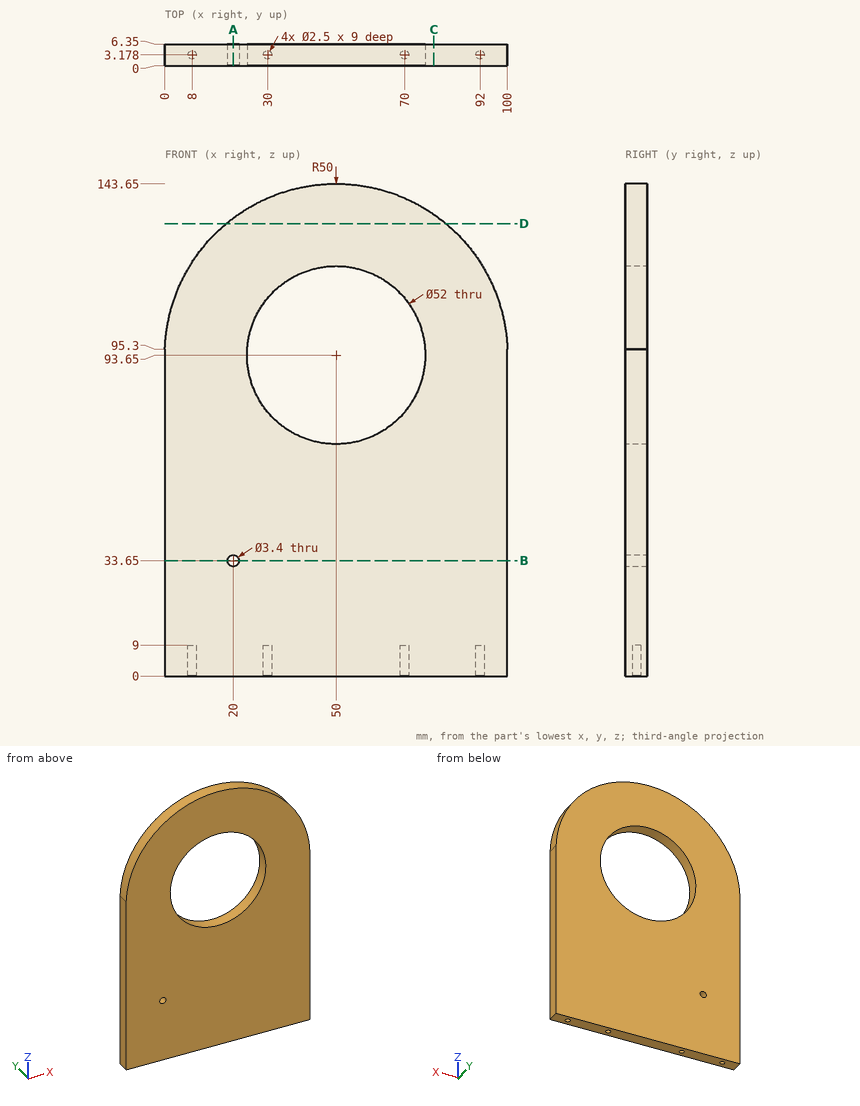
Input: dimensioned drawing with shaded views. Units: mm. Origin: part minimum x, y, z. Round coordinates to 2 decimals unless told otherwise and drop trailing zeros. Loops run counter-clockwise (first coordinate to the right, second up) from the corner with the lowest first, then second, coordinate; pieces in that order, holes last. Notation, with made-up numbers: (-22.5, -20.5) -> (16.5, -20.5) arc R27 ccw to (16.5, 13.5) -> close; hole circle Ø10 at (-13, 69). An arc over 180 degrees is marked (long way). Answer as a JSON object with one key per item and string values. Group by question number.
1) Section query A-A on x = 20. Output: boundary loops of the cut face in (y, z), plus the area to 3 significant figures.
2) Pin query (flat end, axial travel): pin 1 (2 mm diameter, centred on x = 30, y = 3, fed in from -Z); pin 2 (5 mm diameter, centred on x = 35.5, z = 109.5, fed in from -Y); pin 3 (1.5 mm diameter, centred on x = 8, y = 3.18, fed in from +Z) (1 decimal); pin 4 (3 mm diameter, centred on x = 92, y = 3.18, fed in from +Z). Return the tip coordinate at first contact, or that it passes through.
3) Section query D-D on z = 132. Output: boundary loops of the cut face in (x, y).
4) Section query B-B on z = 33.65. Output: boundary loops of the cut face in (x, y).
5) Section query C-C on x = 78.5. Output: boundary loops of the cut face in (y, z).
6) Ray query, L1, parallel to Y at x = 30, z = 5; L2, parallel to X at y = 5, z = 74 (1 decimal); L3, parallel to Z at x = 70, y = 1.5 (1 decimal). Return the intervals inside material, ascending.
Reply:
{
 "1": {"outline": "(0, 0) -> (6.35, 0) -> (6.35, 31.95) -> (0, 31.95) -> close; (0, 35.35) -> (6.35, 35.35) -> (6.35, 133.65) -> (0, 133.65) -> close", "area": "827 mm2"},
 "2": {"pin 1": "stops at z = 9", "pin 2": "passes through", "pin 3": "stops at z = 121.9", "pin 4": "stops at z = 122.97"},
 "3": {"outline": "(17.92, 0) -> (82.08, 0) -> (82.08, 6.35) -> (17.92, 6.35) -> close"},
 "4": {"outline": "(0, 0) -> (18.3, 0) -> (18.3, 6.35) -> (0, 6.35) -> close; (21.7, 0) -> (100, 0) -> (100, 6.35) -> (21.7, 6.35) -> close"},
 "5": {"outline": "(0, 0) -> (6.35, 0) -> (6.35, 134.73) -> (0, 134.73) -> close"},
 "6": {"L1": "y = 0 to 1.93, 4.43 to 6.35", "L2": "x = 0 to 33, 67 to 100", "L3": "z = 0 to 77, 110.3 to 139.5"}
}
